from build123d import *

# Parameters (mm, degrees)
IZIM1_W                     = 80
IZIM1_H                     = 35
Y_KSEKLIK_EKSTR_ZYON1_DEPTH = 35
RADYUS1_R                   = 17.5
RADYUS2_R                   = 17.5
RADYUS3_R                   = 17.5
IZIM2_R                     = 5
KES_EKSTR_ZYON1_DEPTH       = 56.957573214
PAH1_SIZE                   = 10
IZIM3_W                     = 37.5
IZIM3_H                     = 15
Y_KSEKLIK_EKSTR_ZYON2_DEPTH = 5
IZIM4_W                     = 37.5
IZIM4_H                     = 15
Y_KSEKLIK_EKSTR_ZYON3_DEPTH = 5
IZIM6_W                     = 17.989484019
IZIM6_H                     = 35
KES_EKSTR_ZYON2_DEPTH       = 25
IZIM7_W                     = 32.408876432
IZIM7_H                     = 4.5
Y_KSEKLIK_EKSTR_ZYON4_DEPTH = 2.5


# Some blends are built 0.0001 mm under size
with BuildPart() as part:
    # Çizim1 → Yükseklik-Ekstrüzyon1 (new body)
    with BuildSketch(Plane.XY):
        Rectangle(IZIM1_W, IZIM1_H)
    extrude(amount=Y_KSEKLIK_EKSTR_ZYON1_DEPTH)

    # Radyus1
    radyus1_edges = [part.edges().sort_by_distance(p)[0] for p in [
        (-40, 17.5, 17.5),
    ]]
    fillet(radyus1_edges, radius=RADYUS1_R)

    # Radyus2
    radyus2_edges = [part.edges().sort_by_distance(p)[0] for p in [
        (-40, -17.5, 17.5),
    ]]
    fillet(radyus2_edges, radius=RADYUS2_R - 0.0001)  # a hair under: the kernel refuses the full size

    # Radyus3
    radyus3_edges = [part.edges().sort_by_distance(p)[0] for p in [
        (40, -17.5, 17.5),
        (40, 17.5, 17.5),
    ]]
    fillet(radyus3_edges, radius=RADYUS3_R - 0.0001)  # a hair under: the kernel refuses the full size

    # Çizim2 → Kes-Ekstrüzyon1 (cut, through all)
    with BuildSketch(Plane.XY.offset(35)):
        with Locations((-40, 0)):
            Circle(IZIM2_R)
    extrude(amount=-KES_EKSTR_ZYON1_DEPTH, mode=Mode.SUBTRACT)

    # Pah1
    # the kernel refuses this chamfer: 10 mm, written as the material it takes off along each edge
    with BuildSketch(Plane(origin=(48.21692988, -17.5, 0), x_dir=(0, 0.9996219169112968, -0.027495876610586372), z_dir=(-1, 0, 0))) as pah1_piece_1:
        Polygon((PAH1_SIZE * 0.999621916911, -PAH1_SIZE * 0.0274958766106), (-PAH1_SIZE * 0.0274958766106, -PAH1_SIZE * 0.999621916911), (0, 0), align=None)
    extrude(amount=96.433859759, mode=Mode.SUBTRACT)
    with BuildSketch(Plane(origin=(48.21692988, -17.5, 35), x_dir=(0, 0.9996219169112968, 0.027495876610586317), z_dir=(-1, 0, 0))) as pah1_piece_2:
        Polygon((PAH1_SIZE * 0.999621916911, PAH1_SIZE * 0.0274958766106), (-PAH1_SIZE * 0.0274958766106, PAH1_SIZE * 0.999621916911), (0, 0), align=None)
    extrude(amount=96.433859759, mode=Mode.SUBTRACT)
    with BuildSketch(Plane(origin=(-48.21682988, 17.5, 0), x_dir=(0, -0.9996219169112968, -0.027495876610586372), z_dir=(1, 0, 0))) as pah1_piece_3:
        Polygon((PAH1_SIZE * 0.999621916911, -PAH1_SIZE * 0.0274958766106), (-PAH1_SIZE * 0.0274958766106, -PAH1_SIZE * 0.999621916911), (0, 0), align=None)
    extrude(amount=96.433759759, mode=Mode.SUBTRACT)
    with BuildSketch(Plane(origin=(-48.21682988, 17.5, 35), x_dir=(0, -0.9996219169112968, 0.027495876610586317), z_dir=(1, 0, 0))) as pah1_piece_4:
        Polygon((PAH1_SIZE * 0.999621916911, PAH1_SIZE * 0.0274958766106), (-PAH1_SIZE * 0.0274958766106, PAH1_SIZE * 0.999621916911), (0, 0), align=None)
    extrude(amount=96.433759759, mode=Mode.SUBTRACT)

    # Çizim3 → Yükseklik-Ekstrüzyon2 (add)
    with BuildSketch(Plane(origin=(0, 17.5, 0), x_dir=(1, 0, 0), z_dir=(0, 1, 0))):
        with Locations((18.75, -17.5)):
            Rectangle(IZIM3_W, IZIM3_H)
    extrude(amount=-Y_KSEKLIK_EKSTR_ZYON2_DEPTH)

    # Çizim4 → Yükseklik-Ekstrüzyon3 (add)
    with BuildSketch(Plane.XZ.offset(17.5)):
        with Locations((18.75, 17.5)):
            Rectangle(IZIM4_W, IZIM4_H)
    extrude(amount=-Y_KSEKLIK_EKSTR_ZYON3_DEPTH)

    # Çizim6 → Kes-Ekstrüzyon2 (cut)
    with BuildSketch(Plane(origin=(0, -12.5, 0), x_dir=(1, 0, 0), z_dir=(0, 1, 0))):
        with Locations((31.00525799, -17.5)):
            Rectangle(IZIM6_W, IZIM6_H)
    extrude(amount=KES_EKSTR_ZYON2_DEPTH, mode=Mode.SUBTRACT)

    # Çizim7 → Yükseklik-Ekstrüzyon4 (add)
    with BuildSketch(Plane(origin=(37.5, 0, 0), x_dir=(0, 0, -1), z_dir=(1, 0, 0))):
        with Locations((-17.5, 14.75)):
            Rectangle(IZIM7_W, IZIM7_H)
        with Locations((-17.5, -14.75)):
            Rectangle(IZIM7_W, IZIM7_H)
    extrude(amount=Y_KSEKLIK_EKSTR_ZYON4_DEPTH)


solid = part.part
CAD build for the part. Positions are in the model's coordinates, mm. A direction names the side the tool comes from. Round coordinates to 2 decimals unless told otherwise and drop trailing zeros. Write each loop counter-clockwise with the first axis right and the second up, starting at its lowest first coordinate (ties: lowest second). Pieces come first, ordered by that corner, then holes. Notation, with made-up numbers: M 36.25,5 L 51.25,5 A28 cw 51.25,35 Z; hole C 78.5,59 d1. An arc over 180 degrees is marked long. Use a Markdown table: item, result. Add a question column.
1. 3-axis set-ups, long thin cutter, end or side, ignore diameter. For faces 1 (the face through (-1.3, -12.4, 30.1)), 2 (the face through (-2.3, 12.4, 4.9)), 3 (the face through (32.189, 14.573, 8.623)), 4 (the face through (22.011, 0, 18)), 5 (the face through (39, -17, 18)): which of +Z, -Z, +X, -X, +Y, -Y reach the whole face in a straight line?
2. Slice it at B-B on x = -7. Give the cut face in (y, z).
3. Slice it at D-D on z = 23.5. Give the cut face in (x, y).
4. Drill centre lines: probe 1 along Y at (x, z) = (35, 21.5); probe 2 along X at (y, z) = (-13, 28); probe 3 along X at (y, z) = (-15, 29). Where is each one in solid material? Low to high.
5. Slice it at C-C on x = 27. Give the cut face in (y, z).
6. Flat gauge pins, fed straight in: P1, Ø5, axis at y = -13.5, z = 12.5, coming from the -X side; P2, Ø8, axis at y = -8, z = 26.5, coming from the +X side; P3, Ø2, axis at x = 39, y = -15, coming from the +Z side. Where does each tip first touch, or does it go through?
7. Slice it at A-A on z = 6. Give the cut face in (x, y).
Reply:
| question | item | result |
|---|---|---|
| 1 | face 1 | +Z, -X, -Y |
| 1 | face 2 | -Z, -X, +Y |
| 1 | face 3 | -Z, +Y |
| 1 | face 4 | +Z, -Z, +X |
| 1 | face 5 | +Z, -Z, +X, -Y |
| 2 | outline | M -17.5,10 L -7.5,0 L 7.5,0 L 17.5,10 L 17.5,25 L 7.5,35 L -7.5,35 L -17.5,25 Z |
| 3 | outline | M -39.29,-4.95 A17.5 ccw -22.5,-17.5 L 37.5,-17.5 L 37.5,-17 L 40,-17 L 40,-12.5 L 22.01,-12.5 L 22.01,12.5 L 40,12.5 L 40,17 L 37.5,17 L 37.5,17.5 L -22.5,17.5 A17.5 ccw -39.29,4.95 A5 cw Z |
| 4 | probe 1 | y = -17.5 to -12.5, 12.5 to 17.5 |
| 4 | probe 2 | x = -34.22 to 34.22, 37.5 to 40 |
| 4 | probe 3 | x = 37.5 to 40 |
| 5 | outline | M -17.5,10 L -16.91,10 L -16.91,9.41 L -12.5,5 L -12.5,30 L -16.91,25.59 L -16.91,25 L -17.5,25 Z; M 12.5,5 L 16.91,9.41 L 16.91,10 L 17.5,10 L 17.5,25 L 16.91,25 L 16.91,25.59 L 12.5,30 Z |
| 6 | P1 | stops at x = -36.11 |
| 6 | P2 | stops at x = 22.01 |
| 6 | P3 | stops at z = 33.7 |
| 7 | outline | M -39.29,-4.95 A17.5 ccw -33.64,-13.5 L 33.64,-13.5 A17.5 ccw 34.75,-12.5 L 22.01,-12.5 L 22.01,12.5 L 34.75,12.5 A17.5 ccw 33.64,13.5 L -33.64,13.5 A17.5 ccw -39.29,4.95 A5 cw Z; M 37.5,-17 L 40,-17 L 40,-12.5 L 37.5,-12.5 Z; M 37.5,12.5 L 40,12.5 L 40,17 L 37.5,17 Z |
